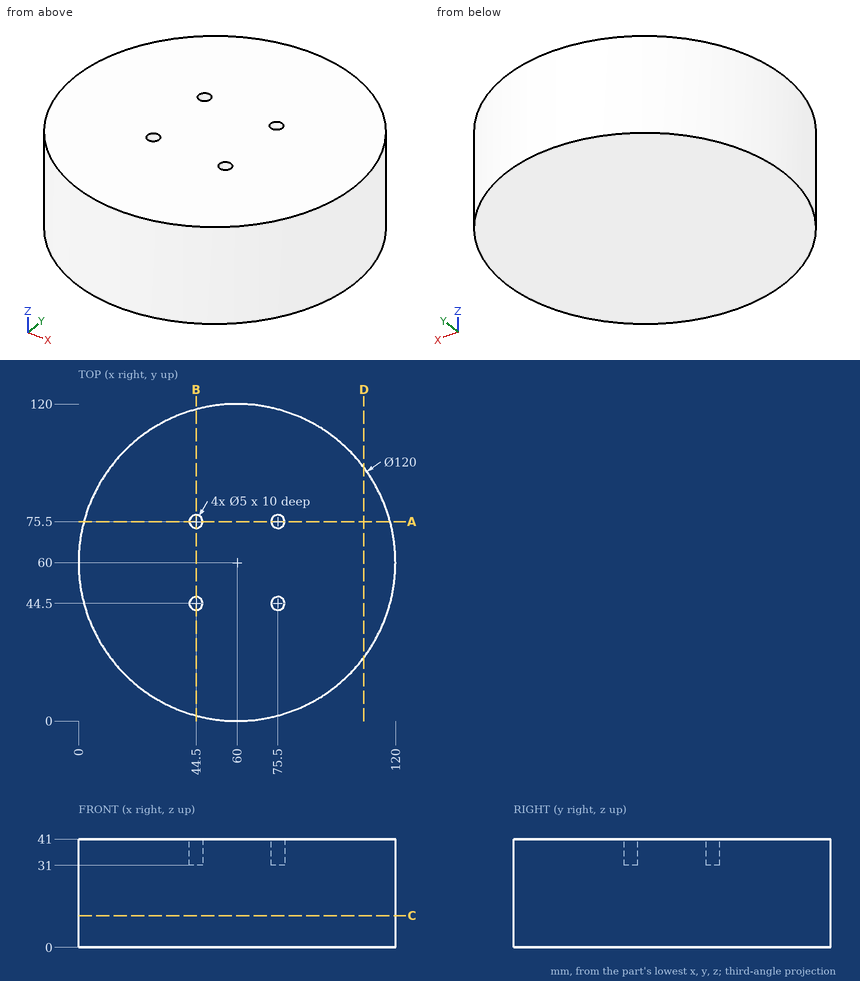
Geometry: see drawing. Coordinates: mm, zero at the bounding-box minimum. Coordinates: 2 decimals unless noted, no trailing zeros. Write each loop counter-clockwise with the first axis right and the second up, starting at its lowest first coordinate (ties: lowest second). Pieces come first, ordered by that corner, then holes.
1) Pin query (flat end, axial travel): pin 1 Ø1 at (y, z) = (83, 7) entering from -X; pin 2 Ø1.5 at (x, y) = (75.5, 44.5) entering from +Z; pin 3 Ø2 at (x, z) = (97.5, 30) entering from -Y. Return the tip coordinate at first contact, or that it passes through.
2) Section A-A on y = 75.5. Output: boundary loops of the cut face in (x, z).
3) Section D-D on x = 108. Output: boundary loops of the cut face in (y, z).
4) Material intervals for line 1 along Y through (x, z) = (75, 33); line 2 along Y through (x, z) = (44, 33); line 3 along X through (y, z) = (75.5, 37.75), sorted ascending.
5) Section C-C on z = 12. Output: boundary loops of the cut face in (x, y), and give its area (3 significant figures).
Check result:
1. pin 1: stops at x = 4.38
1. pin 2: stops at z = 31
1. pin 3: stops at y = 12.38
2. outline: (2.04, 0) - (117.96, 0) - (117.96, 41) - (78, 41) - (78, 31) - (73, 31) - (73, 41) - (47, 41) - (47, 31) - (42, 31) - (42, 41) - (2.04, 41) - close
3. outline: (24, 0) - (96, 0) - (96, 41) - (24, 41) - close
4. line 1: y = 1.91 to 42.05, 46.95 to 73.05, 77.95 to 118.09
4. line 2: y = 2.17 to 42.05, 46.95 to 73.05, 77.95 to 117.83
4. line 3: x = 2.04 to 42, 47 to 73, 78 to 117.96
5. outline: circle Ø120 at (60, 60)
5. area: 11,300 mm2
